from build123d import *

# Parameters (mm, degrees)
SKETCH1_R           = 4.699
BOSS_EXTRUDE3_DEPTH = 1.641793186


with BuildPart() as part:
    # Sketch1 → Boss-Extrude3 (new body)
    with BuildSketch(Plane.XY):
        with BuildLine():
            Line((-46.269533378, 0), (-351.31947646, 0))
            ThreePointArc((-351.31947646, 0), (-368.919381572, -11.759880611), (-364.789860651, -32.520384191))
            Line((-364.789860651, -32.520384191), (-212.125506603, -185.184738239))
            ThreePointArc((-212.125506603, -185.184738239), (-198.655122421, -190.764354058), (-185.184738239, -185.184738239))
            Line((-185.184738239, -185.184738239), (-32.717500753, -32.717500753))
            ThreePointArc((-32.717500753, -32.717500753), (-28.388979015, -11.759100083), (-46.269533378, 0))
        make_face()
        with Locations((-198.655122421, -19.05)):
            Circle(SKETCH1_R, mode=Mode.SUBTRACT)
        with Locations((-279.477427511, -19.05)):
            Circle(SKETCH1_R, mode=Mode.SUBTRACT)
        with Locations((-117.832817213, -19.05)):
            Circle(SKETCH1_R, mode=Mode.SUBTRACT)
        with Locations((-351.319476479, -19.05)):
            Circle(SKETCH1_R, mode=Mode.SUBTRACT)
        with Locations((-45.990768365, -19.05)):
            Circle(SKETCH1_R, mode=Mode.SUBTRACT)
        with Locations((-198.655122421, -171.714354057)):
            Circle(SKETCH1_R, mode=Mode.SUBTRACT)
        with Locations((-162.734097937, -135.793329573)):
            Circle(SKETCH1_R, mode=Mode.SUBTRACT)
        with Locations((-234.576146906, -135.793329573)):
            Circle(SKETCH1_R, mode=Mode.SUBTRACT)
        with Locations((-198.655122421, -99.872305089)):
            Circle(SKETCH1_R, mode=Mode.SUBTRACT)
    extrude(amount=BOSS_EXTRUDE3_DEPTH)


solid = part.part
Geometry: final body of the model. Coordinates: model frame, mm. Coordinates: 2 decimals unless noted, no trailing zeros. Order: outer loops, then holes, each group sorted by start corner. A loop starts at its lowest first (then second) coordinate and runs counter-clockwise, first axis right, second up. Notation, with made-up numbers: M -12.75,-40 L -7.75,-40 A17 cw -7.75,-25 Z; hole C -21,57.25 d1. An arc over 180 degrees is marked long. One line per question, with ' | ' between items. Start each with the question number.
Item 1: Draft query along Y for faces 1 (the flat face through (-289.53, -107.78, 0.81)), 2 (the cylindrical face through (-196.487, -175.883, 0.809)), 3 (the flat face through (-201, -73, 1.642)). Return one class per face: released by +Y, released by -Y, zero draft, split by the parting line, or undercut.
Item 2: Cut plane C-C, the plane x = -100.5. Return the cut outline in (y, z).
Item 3: Pin query (flat end, axial travel): pin 1 Ø10 at (x, y) = (-116.5, -59.5) entering from -Z; pin 2 Ø5.5 at (x, y) = (-198.66, -171.71) entering from +Z. Return the tip coordinate at first contact, or that it passes through.
Item 4: Ray query, probe 1 along X at (y, z) = (-32.5, 0.45); probe 2 along Y at (x, z) = (-164, 0.5); probe 3 along Y at (x, z) = (-46.5, 0.4). Return the intervals inside material, ascending. Write a range as [from, to].
Item 5: Cut plane B-B, the plane z = 1. Count the separate pieces of the cut face and the enclosed holes in it, then the cut area to 3 significant figures.
Item 6: Cut plane D-D, the plane y = -157. Return the cut outline in (x, z).
Item 7: Cut plane A-A, the plane y = -19.05. Return the cut outline in (x, z).
A:
1) face 1: released by -Y | face 2: undercut | face 3: zero draft
2) outline: M -100.5,0 L 0,0 L 0,1.64 L -100.5,1.64 Z
3) pin 1: stops at z = 0 | pin 2: passes through
4) probe 1: x = [-364.81, -32.5] | probe 2: y = [-164, -140.32], [-131.27, 0] | probe 3: y = [-46.5, -23.72], [-14.38, 0]
5) separate pieces: 1 | enclosed holes: 9 | area: 37,900 mm2
6) outline: M -240.31,0 L -157,0 L -157,1.64 L -240.31,1.64 Z
7) outline: M -370.37,0 L -356.02,0 L -356.02,1.64 L -370.37,1.64 Z; M -346.62,0 L -284.18,0 L -284.18,1.64 L -346.62,1.64 Z; M -274.78,0 L -203.35,0 L -203.35,1.64 L -274.78,1.64 Z; M -193.96,0 L -122.53,0 L -122.53,1.64 L -193.96,1.64 Z; M -113.13,0 L -50.69,0 L -50.69,1.64 L -113.13,1.64 Z; M -41.29,0 L -26.94,0 L -26.94,1.64 L -41.29,1.64 Z
